Input: part model. Units: mm. Frame: model coordinates. Coordinates: 2 decimals unless noted, no trailing zeros. Write each loop counter-clockwise with the first axis right and the second up, starting at its lowest first coordinate (ties: lowest second). Pieces come first, ordered by that corner, then holes. Notation, with made-up numbers: M 79.5,-25 L 108.5,-25 A27 cw 108.5,2 Z; hole C 9,-31 d4. An arc over 180 degrees is marked long. Use CSV: the item, a comma, the result in double quotes.
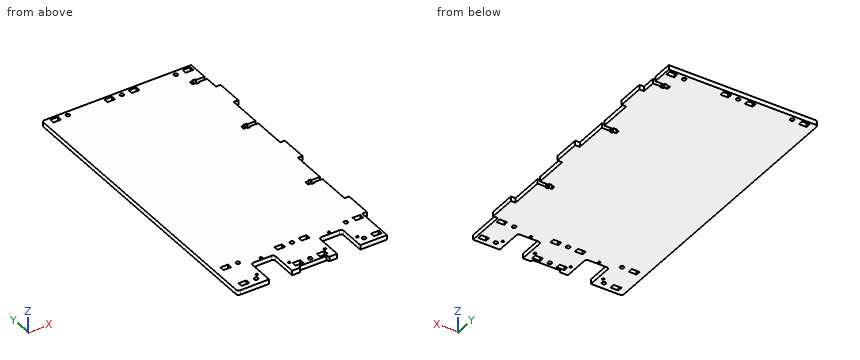
```python
from build123d import *

# Parameters (mm, degrees)
SKETCH_1_R      = 2.5
SKETCH_1_R_2    = 1.5
SKETCH_1_W      = 10
SKETCH_1_H      = 6
EXTRUDE_1_DEPTH = 6
FILLET_1_R      = 3
FILLET_2_R      = 3.5


with BuildPart() as part:
    # Эскиз1 → Бобышка-Вытянуть1 (new body)
    with BuildSketch(Plane.XY):
        Polygon((-100, 9), (-100, -378), (-59.25, -378), (-59.25, -342), (-29.25, -342), (-29.25, -378), (-19.232050808, -378), (-17.5, -375), (17.5, -375), (19.232050808, -378), (29.25, -378), (29.25, -342), (59.25, -342), (59.25, -378), (94, -378), (94, -329), (100, -329), (100, -294), (94, -294), (94, -250.45), (83, -250.45), (83, -251.925), (79.2, -251.925), (79.2, -250.45), (75, -250.45), (75, -245.55), (79.2, -245.55), (79.2, -244.075), (83, -244.075), (83, -245.55), (94, -245.55), (94, -202), (100, -202), (100, -167), (94, -167), (94, -123.45), (83, -123.45), (83, -124.925), (79.2, -124.925), (79.2, -123.45), (75, -123.45), (75, -118.55), (79.2, -118.55), (79.2, -117.075), (83, -117.075), (83, -118.55), (94, -118.55), (94, -75), (100, -75), (100, -40), (94, -40), (94, -22.45), (83, -22.45), (83, -23.925), (79.2, -23.925), (79.2, -22.45), (75, -22.45), (75, -17.55), (79.2, -17.55), (79.2, -16.075), (83, -16.075), (83, -17.55), (94, -17.55), (94, 9), align=None)
        with Locations((-70.1375, 3)):
            Circle(SKETCH_1_R, mode=Mode.SUBTRACT)
        with Locations((0, 3)):
            Circle(SKETCH_1_R, mode=Mode.SUBTRACT)
        with Locations(Location((70.1375, 3, 0), (0, 0, 180))):
            Circle(SKETCH_1_R, mode=Mode.SUBTRACT)
        with Locations((-70.1375, -333)):
            Circle(SKETCH_1_R, mode=Mode.SUBTRACT)
        with Locations((0, -333)):
            Circle(SKETCH_1_R, mode=Mode.SUBTRACT)
        with Locations(Location((70.1375, -333, 0), (0, 0, 180))):
            Circle(SKETCH_1_R, mode=Mode.SUBTRACT)
        with Locations((-70.1375, -369)):
            Circle(SKETCH_1_R, mode=Mode.SUBTRACT)
        with Locations((0, -369)):
            Circle(SKETCH_1_R, mode=Mode.SUBTRACT)
        with Locations(Location((70.1375, -369, 0), (0, 0, 180))):
            Circle(SKETCH_1_R, mode=Mode.SUBTRACT)
        with Locations((-65.25, -363)):
            Circle(SKETCH_1_R_2, mode=Mode.SUBTRACT)
        with Locations((-44.25, -339)):
            Circle(SKETCH_1_R_2, mode=Mode.SUBTRACT)
        with Locations(Location((-23.25, -363, 0), (0, 0, 180))):
            Circle(SKETCH_1_R_2, mode=Mode.SUBTRACT)
        with Locations((23.25, -363)):
            Circle(SKETCH_1_R_2, mode=Mode.SUBTRACT)
        with Locations(Location((44.25, -339, 0), (0, 0, 180))):
            Circle(SKETCH_1_R_2, mode=Mode.SUBTRACT)
        with Locations(Location((65.25, -363, 0), (0, 0, 180))):
            Circle(SKETCH_1_R_2, mode=Mode.SUBTRACT)
        with Locations((86, 3)):
            Rectangle(SKETCH_1_W, SKETCH_1_H, mode=Mode.SUBTRACT)
        with Locations((15.8625, 3)):
            Rectangle(SKETCH_1_W, SKETCH_1_H, mode=Mode.SUBTRACT)
        with Locations((-15.8625, 3)):
            Rectangle(SKETCH_1_W, SKETCH_1_H, mode=Mode.SUBTRACT)
        with Locations((-86, 3)):
            Rectangle(SKETCH_1_W, SKETCH_1_H, mode=Mode.SUBTRACT)
        with Locations((86, -333)):
            Rectangle(SKETCH_1_W, SKETCH_1_H, mode=Mode.SUBTRACT)
        with Locations((15.8625, -333)):
            Rectangle(SKETCH_1_W, SKETCH_1_H, mode=Mode.SUBTRACT)
        with Locations((-15.8625, -333)):
            Rectangle(SKETCH_1_W, SKETCH_1_H, mode=Mode.SUBTRACT)
        with Locations((-86, -333)):
            Rectangle(SKETCH_1_W, SKETCH_1_H, mode=Mode.SUBTRACT)
        with Locations((86, -369)):
            Rectangle(SKETCH_1_W, SKETCH_1_H, mode=Mode.SUBTRACT)
        with Locations((15.8625, -369)):
            Rectangle(SKETCH_1_W, SKETCH_1_H, mode=Mode.SUBTRACT)
        with Locations((-15.8625, -369)):
            Rectangle(SKETCH_1_W, SKETCH_1_H, mode=Mode.SUBTRACT)
        with Locations((-86, -369)):
            Rectangle(SKETCH_1_W, SKETCH_1_H, mode=Mode.SUBTRACT)
    extrude(amount=EXTRUDE_1_DEPTH)

    # Скругление1
    fillet_1_edges = [part.edges().sort_by_distance(p)[0] for p in [
        (59.25, -342, 3),
        (29.25, -342, 3),
        (-29.25, -342, 3),
        (-59.25, -342, 3),
        (-100, 9, 3),
    ]]
    fillet(fillet_1_edges, radius=FILLET_1_R)

    # Скругление2
    fillet_2_edges = [part.edges().sort_by_distance(p)[0] for p in [
        (-100, -378, 3),
    ]]
    fillet(fillet_2_edges, radius=FILLET_2_R)


solid = part.part
```
1. Contact query for flat-ended pins moving along their axis: pin 1 Ø1.8 at (y, z) = (-348.5, 4.5) entering from +X; pin 2 Ø3 at (x, z) = (18, 2.5) entering from -Y. Output: stop coordinate, or through.
Resolved:
pin 1,"stops at x = 94"
pin 2,"stops at y = -378"
2. Section B-B (y = -265). Return loops of the section in (x, z), then the cut area to 3 significant figures.
Resolved:
outline,"M -100,0 L 94,0 L 94,6 L -100,6 Z"
area,"1,160 mm^2"
3. Section A-A (z = 4.35). State how many separate pieces and enclosed holes the cut face has, then the cut area to 3 significant figures.
Resolved:
separate pieces,"1"
enclosed holes,"27"
area,"72,200 mm^2"
4. Material intervals for line 1 (Y direction, x = -12.5, z = 1.4); line 2 (Y direction, x = -83, z = 2.4); line 3 (Y direction, x = -23.5, z = 4.75), sorted ascending. Write a range as [from, to].
Resolved:
line 1,"y = [-375, -372], [-366, -336], [-330, 0], [6, 9]"
line 2,"y = [-378, -372], [-366, -336], [-330, 0], [6, 9]"
line 3,"y = [-378, -364.48], [-361.52, 9]"
